Job drawing, mm, ordinate dimensions from the low corner. One solid piece. A direction names the side the tool comes from. Round coordinates to 2 decimals unless told otherwise and drop trailing zeros. Order: outer loops, then holes, each group sorted by start corner. A loop starts at its lowest first (then second) coordinate and runs counter-clockwise, first axis right, second up. Notation, with made-up numbers: (66.5, 26.5) -> (98.5, 26.5) arc R29 ccw to (98.5, 58.5) -> close; hole circle Ø1 at (-40, 28). An arc over 180 degrees is marked (long way). Write item = value, one per line.
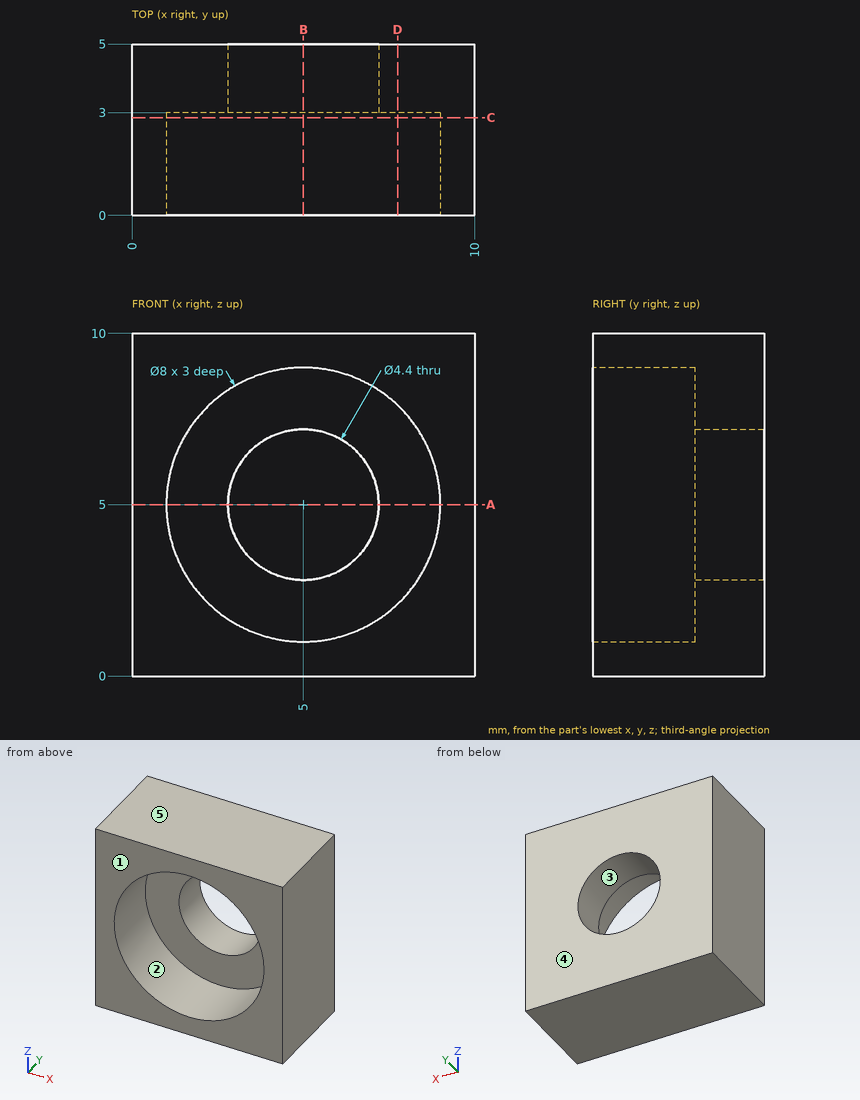
Q1. Cut at B-B, the plane x = 5. List the corners of the cut face in (y, z).
Check values:
outline = (0, 0) -> (5, 0) -> (5, 2.8) -> (3, 2.8) -> (3, 1) -> (0, 1) -> close; (0, 9) -> (3, 9) -> (3, 7.2) -> (5, 7.2) -> (5, 10) -> (0, 10) -> close
Q2. Cut at C-C, the plane y = 2.85. List the corners of the cut face in (x, z), and give its area (3 significant figures).
Check values:
outline = (0, 0) -> (10, 0) -> (10, 10) -> (0, 10) -> close; hole circle Ø8 at (5, 5)
area = 49.7 mm²
Q3. Mould opens along Z. For the marked faces 3, 4 and 5 say: released by +Z, released by -Z, zero draft, split by the parting line, or undercut.
Check values:
face_3 = undercut
face_4 = zero draft
face_5 = released by +Z
Q4. Cut at A-A, the plane z = 5. List the corners of the cut face in (x, y).
Check values:
outline = (0, 0) -> (1, 0) -> (1, 3) -> (2.8, 3) -> (2.8, 5) -> (0, 5) -> close; (7.2, 3) -> (9, 3) -> (9, 0) -> (10, 0) -> (10, 5) -> (7.2, 5) -> close
Q5. Flat gauge pin, fed straight in: pin 1 (1.5 mm diameter, centred on x = 5, z = 5, fed in from -Y). Where does the tip first touch, or does it go through?
Check values:
pin_1 = through
Q6. Which spindle directions (+Z, -Z, +X, -X, +Y, -Y) get a long thin tool onto all of the face, cutting with end or side? Do the marked faces 1 and 2. Say none if no direction does.
Check values:
face_1 = +Z, -Z, +X, -X, -Y
face_2 = -Y
Q7. Probe probe 1 along X at (y, z) = (1.5, 5); probe 2 along Z at (x, y) = (5, 3.75). List the from-to ranges inside material, lowest first.
Check values:
probe_1 = 0 to 1, 9 to 10
probe_2 = 0 to 2.8, 7.2 to 10
Q8. Cut at D-D, the plane x = 7.75. List the corners of the cut face in (y, z), and give its area (3 significant figures).
Check values:
outline = (0, 0) -> (5, 0) -> (5, 10) -> (0, 10) -> (0, 7.9) -> (3, 7.9) -> (3, 2.1) -> (0, 2.1) -> close
area = 32.6 mm²
